Source: CAD feature listing. Evaluate the final solid. Frame: model axes, mm. A direction names the side the tool comes from. Coordinates: 2 decimals unless noted, no trailing zeros. Write each loop counter-clockwise with the first axis right and the second up, starting at its lowest first coordinate (ties: lowest second). Pieces come first, ordered by that corner, then holes. Notation, with made-up numbers: (31, 75.25) -> (57, 75.25) arc R29 cw to (57, 104.25) -> close; hole circle Ø2 at (39, -13). An arc over 180 degrees is marked (long way). One line per item, written item: value. Start each with the question number.
1. Mould query, pull axis Z, two halves, no side actions, for faces 1 (the flat face through (-1, 6.35, 13)), 2 (the cylindrical face through (1.38, 3.13, 6.2)), 3 (the cylindrical face through (-13.35, 4.78, 60.13)). Classes: released by +Z, released by -Z, zero draft, split by the parting line, or undercut.
2. Line query: line 1 (Z direction, x = 0, y = 3.25) (3 decimals); line 2 (X direction, y = 1, z = -39); line 3 (X direction, y = 5, z = 35). Output: solid intervals per line, ascending.
3. Section query B-B, the plane z = 0. Output: boundary loops of the cut face in (x, y) (3 decimals).
4. Access query for faces 4 (the flat face through (58, 3.175, 24)), 5 (the cylindrical face through (-14.18, 1.57, 63.85)), 6 (the cylindrical face through (-34.984, 0.783, 27.787)). Directions: +Z, -Z, +X, -X, +Y, -Y. A direction counts if a zero-diameter tool reaches every point of the face in a straight line with its end or side. Return the directions, or none.
5. Section query D-D, the plane z = -24.5. Output: boundary loops of the cut face in (x, y) (3 decimals), and give its area (3 significant figures).
6. Section query A-A, the plane x = 0. Output: boundary loops of the cut face in (y, z) (3 decimals), and give its area (3 significant figures).
7. Section query C-C, the plane x = 35. State how many separate pieces and enclosed holes the cut face has, and give its area (3 significant figures).
8. First-contact query: P1, Ø9.5, axis at x = -31, z = -34, coming from the -Y side; P2, Ø3.5, axis at x = -30.5, z = 36, coming from the -Y side; P3, Ø2, axis at y = 3.5, z = 26, coming from the +X side. Flat tips, straight axial feed; report the tip coordinate or a pass-through.
from build123d import *

# Parameters (mm, degrees)
SKETCH2_R                   = 65.405
BOSS_EXTRUDE1_DEPTH         = 6.35
SKETCH4_R                   = 65.405
SKETCH4_R_2                 = 61.595
CUT_EXTRUDE1_DEPTH          = 3.175
F_1_4_0_25_DIAMETER_HOLE1_D = 6.35
F_1_2_0_5_DIAMETER_HOLE1_D  = 12.7
SKETCH9_R                   = 6.0325
CUT_EXTRUDE2_DEPTH          = 1.5875


with BuildPart() as part:
    # Sketch2 → Boss-Extrude1 (new body)
    with BuildSketch(Plane(origin=(0, 0, 0), x_dir=(1, 0, 0), z_dir=(0, 1, 0))):
        Circle(SKETCH2_R)
    extrude(amount=BOSS_EXTRUDE1_DEPTH)

    # Sketch4 → Cut-Extrude1 (cut)
    with BuildSketch(Plane(origin=(0, 6.35, 0), x_dir=(1, 0, 0), z_dir=(0, 1, 0))):
        Circle(SKETCH4_R)
        Circle(SKETCH4_R_2, mode=Mode.SUBTRACT)
    extrude(amount=-CUT_EXTRUDE1_DEPTH, mode=Mode.SUBTRACT)

    # 1/4 (0.25) Diameter Hole1 (through all)
    with Locations(Plane(origin=(0, 6.35, 0), x_dir=(1, 0, 0), z_dir=(0, 1, 0))):
        with Locations((-33.675960454, 33.675960454), (-33.675960454, -33.675960454), (33.675960454, 33.675960454), (33.675960454, -33.675960454)):
            Hole(F_1_4_0_25_DIAMETER_HOLE1_D / 2)

    # 1/2 (0.5) Diameter Hole1 (through all)
    with Locations(Plane(origin=(0, 6.35, 0), x_dir=(1, 0, 0), z_dir=(0, 1, 0))):
        with Locations((0, 0)):
            Hole(F_1_2_0_5_DIAMETER_HOLE1_D / 2)

    # Sketch9 → Cut-Extrude2 (cut)
    with BuildSketch(Plane.XZ):
        with Locations((-33.675960454, 33.675960454)):
            Circle(SKETCH9_R)
        with Locations((33.675960454, 33.675960454)):
            Circle(SKETCH9_R)
        with Locations((33.675960454, -33.675960454)):
            Circle(SKETCH9_R)
        with Locations((-33.675960454, -33.675960454)):
            Circle(SKETCH9_R)
    extrude(amount=-CUT_EXTRUDE2_DEPTH, mode=Mode.SUBTRACT)


solid = part.part
Computed values:
1. face 1: zero draft
1. face 2: undercut
1. face 3: split by the parting line
2. line 1: z = -61.595 to -6.35, 6.35 to 61.595
2. line 2: x = -52.51 to -36.51, -30.84 to 30.84, 36.51 to 52.51
2. line 3: x = -50.68 to -36.56, -30.79 to 30.79, 36.56 to 50.68
3. outline: (-65.405, 0) -> (-6.35, 0) -> (-6.35, 6.35) -> (-61.595, 6.35) -> (-61.595, 3.175) -> (-65.405, 3.175) -> close; (6.35, 0) -> (65.405, 0) -> (65.405, 3.175) -> (61.595, 3.175) -> (61.595, 6.35) -> (6.35, 6.35) -> close
4. face 4: +Y
4. face 5: +Y, -Y
4. face 6: -Y
5. outline: (-60.643, 0) -> (60.643, 0) -> (60.643, 3.175) -> (56.513, 3.175) -> (56.513, 6.35) -> (-56.513, 6.35) -> (-56.513, 3.175) -> (-60.643, 3.175) -> close
5. area: 744 mm²
6. outline: (0, -65.405) -> (3.175, -65.405) -> (3.175, -61.595) -> (6.35, -61.595) -> (6.35, -6.35) -> (0, -6.35) -> close; (0, 6.35) -> (6.35, 6.35) -> (6.35, 61.595) -> (3.175, 61.595) -> (3.175, 65.405) -> (0, 65.405) -> close
6. area: 726 mm²
7. separate pieces: 3
7. enclosed holes: 0
7. area: 580 mm²
8. P1: stops at y = 0
8. P2: stops at y = 1.59
8. P3: stops at x = 60.42
